Here's how the part is built. I have some questions about the finished solid (model axes, mm). Face numbers are marked on the shaded views. Coordinates: 2 decimals unless noted, no trailing zeros. Write each loop counter-clockwise with the first axis right and the second up, starting at its lowest first coordinate (ties: lowest second). Pieces come first, ordered by that corner, then holes.
```python
from build123d import *

# Parameters (mm, degrees)
F0_W     = 60
F0_H     = 130
F1_DEPTH = 9
F2_R     = 5
F3_R     = 5
F4_R     = 5
F5_R     = 5
F6_R     = 5.5
F7_DEPTH = 0.4
F8_R     = 0.39999


# Not quite as in the source:
# - a fillet or chamfer is up to 0.001 mm smaller than in the source, because OpenCascade refuses the exact size


with BuildPart() as f1:
    # F0 (on Top) → F1 (new body)
    with BuildSketch(Plane.XY):
        with Locations((-13.6178402903, -1.0656192899)):
            Rectangle(F0_W, F0_H)
    extrude(amount=F1_DEPTH)

    # F2
    f2_edges = [f1.edges().sort_by_distance(p)[0] for p in [
        (16.38216, -1.065619, 0),
    ]]
    fillet(f2_edges, radius=F2_R)

    # F3
    f3_edges = [f1.edges().sort_by_distance(p)[0] for p in [
        (-43.61784, -1.065619, 0),
    ]]
    fillet(f3_edges, radius=F3_R)

    # F4
    f4_edges = [f1.edges().sort_by_distance(p)[0] for p in [
        (-13.61784, 63.934381, 0),
    ]]
    fillet(f4_edges, radius=F4_R)

    # F5
    f5_edges = [f1.edges().sort_by_distance(p)[0] for p in [
        (-13.61784, -66.065619, 0),
    ]]
    fillet(f5_edges, radius=F5_R)

    # F6 (on face) → F7 (cut)
    with BuildSketch(Plane.XY.offset(9)):
        with Locations((-15.1178402903, -57.5656192899)):
            Circle(F6_R)
    extrude(amount=-F7_DEPTH, mode=Mode.SUBTRACT)

    # F8 (radius 0.4 in the source; OpenCascade refuses exactly that, so slightly less here)
    f8_edges = [f1.edges().sort_by_distance(p)[0] for p in [
        (-20.61784, -57.565619, 8.6),
    ]]
    fillet(f8_edges, radius=F8_R)


solid = f1.part
```
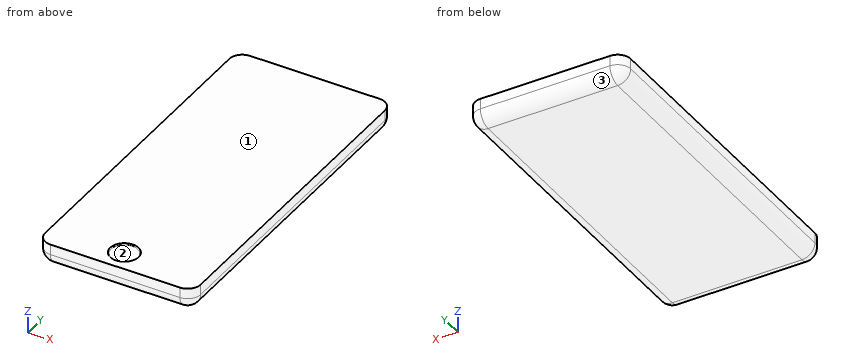
1) We'd pull the mould along Y, two halves only. Please class the marked faces 1, 2 and 3: pulls with the +Y half, pulls with the -Y half, needs draft (parallel to the pull), parting line crosses it, or undercut.
Values follow:
face 1: needs draft
face 2: undercut
face 3: pulls with the +Y half
2) I need wall thicknesses on probe 1 along Y at (x, z) = (-16.5, 4.5); probe 2 along Z at (x, y) = (-39, 10); probe 3 along Y at (x, z) = (-39, 5.5). Which ranges of each line are inside material? Lowest first, please.
Values follow:
probe 1: y = -66.04 to 63.91
probe 2: z = 0.01 to 9
probe 3: y = -66.05 to 63.92
3) Imagine slicing it at A-A on y = -45.5. Please give me the cut outline in (x, z).
Values follow:
outline: (-43.62, 5) arc R5 ccw to (-38.62, 0) - (11.38, 0) arc R5 ccw to (16.38, 5) - (16.38, 9) - (-43.62, 9) - close
4) Imagine slicing it at B-B on z = 1.5. Please give me the cut outline in (x, y), then the cut area to 3 significant figures.
Values follow:
outline: (-42.19, -61.07) arc R3.57 ccw to (-38.62, -64.64) - (11.38, -64.64) arc R3.57 ccw to (14.95, -61.07) - (14.95, 58.93) arc R3.57 ccw to (11.38, 62.51) - (-38.62, 62.51) arc R3.57 ccw to (-42.19, 58.93) - close
area: 7,250 mm2
